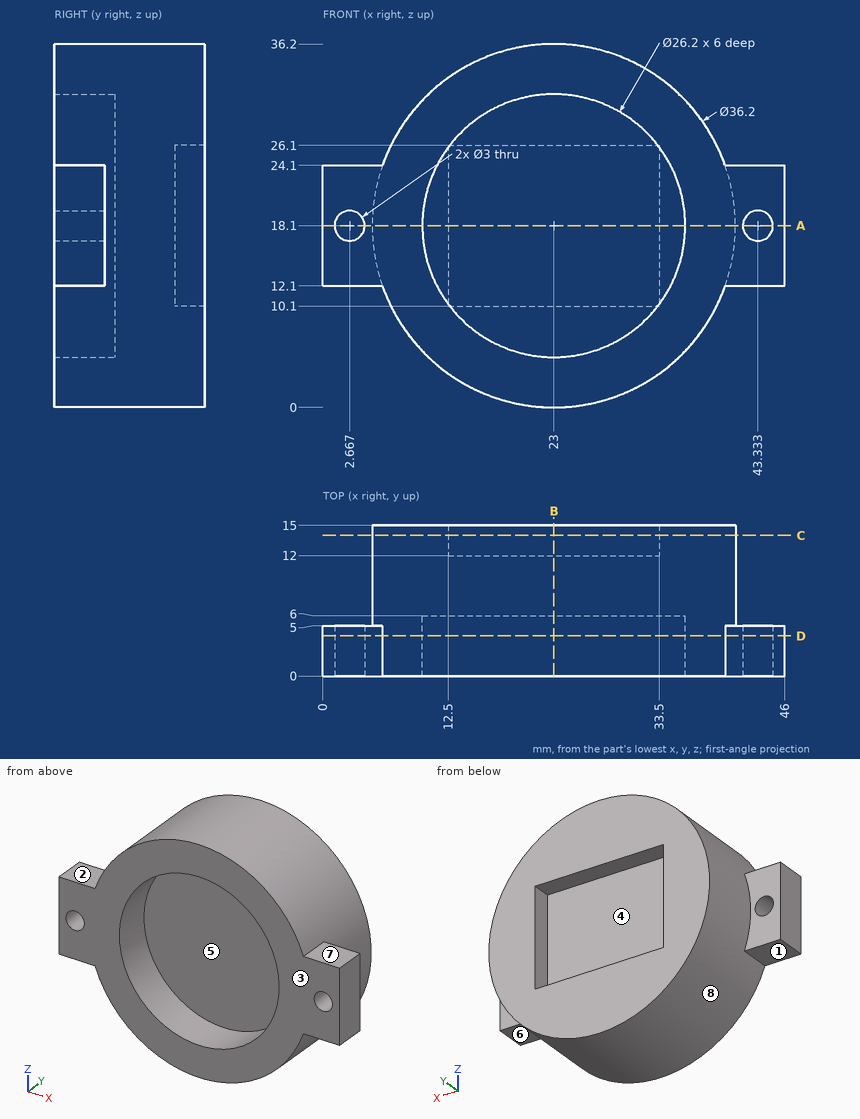
Here's the drawing with two shaded views (mm, measured from the low corner). I have some questions. A direction names the side the tool comes from. Round coordinates to 2 decimals unless told otherwise and drop trailing zeros. Loops run counter-clockwise (first coordinate to the right, second up) from the corner with the lowest first, then second, coordinate; pieces in that order, holes last.
Item 1: If we mould it in two halves opening along Z, with no side actions, what happens to the marked faces 1, 2, 3 and 4? For each: +Z half, -Z half, draft (parallel to the pull), parting line (faces both ways), or undercut.
Item 2: Which directions (+Z, -Z, +X, -X, +Y, -Y) give clear straight access to the entire face, cutting with the end or side of a thin tool? Please do the marked faces 5, 6, 7 and 8.
Item 3: Suppose I cut it at C-C, the plane y = 14. Write out the boundary of the cut face in (x, z), then the cut area to 3 significant figures.
Item 4: Will these pins go through, and if not, where does the flat tip stop? pin 1 Ø2 at (x, y) = (13.5, 12) entering from -Z; pin 2 Ø2.5 at (x, y) = (27.5, 14) entering from -Z; pin 3 Ø2.5 at (x, y) = (41.5, 2) entering from +Z.
Item 5: Please list where these lines run through material, in increasing order: L1, parallel to X at y = 4.05, z = 18.1; L2, parallel to Y at x = 23, z = 20.5; L3, parallel to Z at x = 21.5, y = 13.75.
Item 6: Suppose I cut it at B-B, the plane x = 23. Write out the boundary of the cut face in (y, z), then the cut area to 3 significant figures.
Item 7: Suppose I cut it at D-D, the plane y = 4. Write out the boundary of the cut face in (x, z).
Item 8: Suppose I cut it at A-A, the plane z = 18.1. Write out the boundary of the cut face in (x, y).
Reported:
1. face 1: -Z half
1. face 2: +Z half
1. face 3: draft
1. face 4: undercut
2. face 5: -Y
2. face 6: -Z, +X, +Y, -Y
2. face 7: +Z, +X, +Y, -Y
2. face 8: +Y
3. outline: circle Ø36.2 at (23, 18.1); hole (12.5, 10.1) - (33.5, 10.1) - (33.5, 26.1) - (12.5, 26.1) - close
3. area: 693 mm2
4. pin 1: stops at z = 2.12
4. pin 2: stops at z = 0.29
4. pin 3: stops at z = 24.1
5. L1: x = 0 to 1.17, 4.17 to 9.9, 36.1 to 41.83, 44.83 to 46
5. L2: y = 6 to 12
5. L3: z = 0.06 to 10.1, 26.1 to 36.14
6. outline: (0, 0) - (15, 0) - (15, 10.1) - (12, 10.1) - (12, 26.1) - (15, 26.1) - (15, 36.2) - (0, 36.2) - (0, 31.2) - (6, 31.2) - (6, 5) - (0, 5) - close
6. area: 338 mm2
7. outline: (0, 12.1) - (5.92, 12.1) arc R18.1 ccw to (40.08, 12.1) - (46, 12.1) - (46, 24.1) - (40.08, 24.1) arc R18.1 ccw to (5.92, 24.1) - (0, 24.1) - close; hole circle Ø3 at (2.67, 18.1); hole circle Ø26.2 at (23, 18.1); hole circle Ø3 at (43.33, 18.1)
8. outline: (0, 0) - (1.17, 0) - (1.17, 5) - (0, 5) - close; (4.17, 0) - (9.9, 0) - (9.9, 6) - (36.1, 6) - (36.1, 0) - (41.83, 0) - (41.83, 5) - (41.1, 5) - (41.1, 15) - (33.5, 15) - (33.5, 12) - (12.5, 12) - (12.5, 15) - (4.9, 15) - (4.9, 5) - (4.17, 5) - close; (44.83, 0) - (46, 0) - (46, 5) - (44.83, 5) - close
